Source: three-view drawing plus pictorial views. Frame: mm from the lowest corner of the part. A direction names the side the tool comes from. Give positions to 0.01 mm unless a question says otherwise; leave off trailing zeros. Order: outer loops, then holes, each group sorted by start corner. A loop starts at its lowest first (then second) coordinate and runs counter-clockwise, first axis right, second up. Notation, with made-up numbers: (1.5, 34) -> (21.5, 34) arc R29 cw to (21.5, 54) -> close; hole circle Ø7 at (88.5, -6.5). An arc over 180 degrees is marked (long way). One line per question, with ' | ' between items.
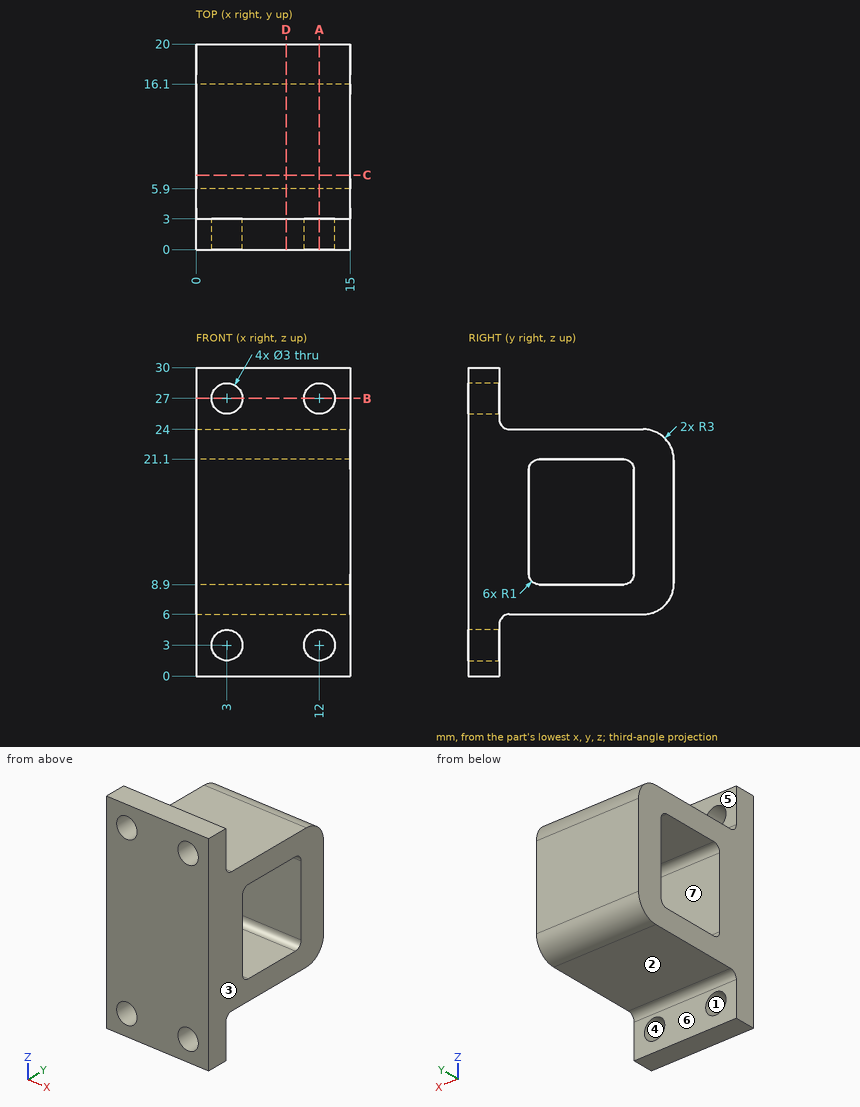
1) Section A-A on x = 12. Return loops of the section in (y, z).
Check result:
outline: (0, 0) -> (3, 0) -> (3, 1.5) -> (0, 1.5) -> close; (0, 4.5) -> (3, 4.5) -> (3, 5) arc R1 cw to (4, 6) -> (17, 6) arc R3 ccw to (20, 9) -> (20, 21) arc R3 ccw to (17, 24) -> (4, 24) arc R1 cw to (3, 25) -> (3, 25.5) -> (0, 25.5) -> close; (0, 28.5) -> (3, 28.5) -> (3, 30) -> (0, 30) -> close; hole (5.9, 9.9) arc R1 ccw to (6.9, 8.9) -> (15.1, 8.9) arc R1 ccw to (16.1, 9.9) -> (16.1, 20.1) arc R1 ccw to (15.1, 21.1) -> (6.9, 21.1) arc R1 ccw to (5.9, 20.1) -> close
2) Set-up query: the marked faces 4, 5, 6 and 7. Return all of +Z, -Z, +X, -X, +Y, -Y with unobstructed straight access to the full face (end or side cutting, diameter ignored); none if empty.
Check result:
face 4: +Y, -Y | face 5: +Z, +X, -X, +Y | face 6: -Z, +X, -X, +Y | face 7: +X, -X
3) Section C-C on y = 7.25. Return loops of the section in (x, z), plus the area to 3 significant figures.
Check result:
outline: (0, 6) -> (15, 6) -> (15, 8.9) -> (0, 8.9) -> close; (0, 21.1) -> (15, 21.1) -> (15, 24) -> (0, 24) -> close | area: 87.0 mm^2
4) Material intervals for probe 1 along X at (y, z) = (1.3, 27); probe 2 along Y at (x, z) = (14, 12.5); probe 3 along Z at (x, y) = (9, 9), sorted ascending. Write a range as from..to.
Check result:
probe 1: x = 0..1.5, 4.5..10.5, 13.5..15 | probe 2: y = 0..5.9, 16.1..20 | probe 3: z = 6..8.9, 21.1..24
5) Contact query for flat-ended pins moving along their axis: pin 1 Ø6 at (x, z) = (6.5, 5) entering from -Y; pin 2 Ø4 at (x, z) = (9, 28) entering from +Y; pin 3 Ø1.5 at (y, z) = (14.5, 4) entering from +X; pin 4 Ø3 at (x, z) = (6.5, 7) entering from +Y. Output: stop coordinate, or through.
Check result:
pin 1: stops at y = 0 | pin 2: stops at y = 3 | pin 3: passes through | pin 4: stops at y = 19.96
6) Section B-B on z = 27. Return loops of the section in (x, y).
Check result:
outline: (0, 0) -> (1.5, 0) -> (1.5, 3) -> (0, 3) -> close; (4.5, 0) -> (10.5, 0) -> (10.5, 3) -> (4.5, 3) -> close; (13.5, 0) -> (15, 0) -> (15, 3) -> (13.5, 3) -> close
7) Section D-D on x = 8.75. Return loops of the section in (y, z), plus the area to 3 significant figures.
Check result:
outline: (0, 0) -> (3, 0) -> (3, 5) arc R1 cw to (4, 6) -> (17, 6) arc R3 ccw to (20, 9) -> (20, 21) arc R3 ccw to (17, 24) -> (4, 24) arc R1 cw to (3, 25) -> (3, 30) -> (0, 30) -> close; hole (5.9, 9.9) arc R1 ccw to (6.9, 8.9) -> (15.1, 8.9) arc R1 ccw to (16.1, 9.9) -> (16.1, 20.1) arc R1 ccw to (15.1, 21.1) -> (6.9, 21.1) arc R1 ccw to (5.9, 20.1) -> close | area: 269 mm^2
8) Pull-direction query (X, two-part tool) for the marked faces 1, 2 and 3; classes: +X half, -X half, draft (parallel to the pull), parting line (faces both ways), or undercut.
Check result:
face 1: undercut | face 2: draft | face 3: +X half
